```python
from build123d import *

# Parameters (mm, degrees)
SKETCH1_W              = 34
SKETCH1_H              = 150
BOSS_EXTRUDE1_DEPTH    = 6.35
SKETCH3_W              = 30
SKETCH3_H              = 6.35
BOSS_EXTRUDE2_DEPTH    = 6.35
F_8_CLEARANCE_HOLE1_D  = 4.3053
F_10_CLEARANCE_HOLE1_D = 4.9784


with BuildPart() as part:
    # Sketch1 → Boss-Extrude1 (new body)
    with BuildSketch(Plane.XY):
        Rectangle(SKETCH1_W, SKETCH1_H)
    extrude(amount=BOSS_EXTRUDE1_DEPTH)

    # Sketch3 → Boss-Extrude2 (add)
    with BuildSketch(Plane.XY.offset(6.35)):
        with Locations((0, 78.175)):
            Rectangle(SKETCH3_W, SKETCH3_H)
        with Locations((0, -78.175)):
            Rectangle(SKETCH3_W, SKETCH3_H)
    extrude(amount=-BOSS_EXTRUDE2_DEPTH)

    # #8 Clearance Hole1 (through all)
    with Locations(Plane.XY.offset(6.35)):
        with Locations((-8, 59.5), (8, 59.5), (8, 35.5), (-8, 35.5), (-8, -35.5), (-8, -59.5), (8, -59.5), (8, -35.5)):
            Hole(F_8_CLEARANCE_HOLE1_D / 2)

    # #10 Clearance Hole1 (through all)
    with Locations(Plane.XY.offset(6.35)):
        with Locations((-6.5, 10), (-6.5, -10)):
            Hole(F_10_CLEARANCE_HOLE1_D / 2)


solid = part.part
```
Work out the finished part from the listing and answer in its coordinate system (mm). A direction names the side the tool comes from. Round coordinates to 2 decimals unless told otherwise and drop trailing zeros. Write each loop counter-clockwise with the first axis right and the second up, starting at its lowest first coordinate (ties: lowest second). Pieces come first, ordered by that corner, then holes. Notation, with made-up numbers: (45.5, 52.5) -> (58.5, 52.5) arc R11 cw to (58.5, 57.5) -> close; hole circle Ø2 at (39, 60.25). An arc over 180 degrees is marked (long way). Write each question's results on one line, items separated by ' | '.
1) Which of the six approach directions +Z, -Z, +X, -X, +Y, -Y give full straight-line access (tool end or side, diameter ignored) to faces 1 (the flat face through (0, 1, 6.35)), 2 (the flat face through (-15, 78, 3)), 3 (the flat face through (15, -78, 3))?
Findings:
face 1: +Z, +X, -X, +Y, -Y | face 2: +Z, -Z, -X, +Y | face 3: +Z, -Z, +X, -Y
2) For a pull along X with two mould halves and no side action, classify faces 4 (the flat face through (15, 78, 3)), 5 (the flat face through (-15, -78, 3)), 6 (the cylindrical face through (5.947, -34.853, 3.131)), 7 (the flat face through (0, -81.35, 3)) as +X half, -X half, draft (parallel to the pull), parting line (faces both ways), or undercut.
Findings:
face 4: +X half | face 5: -X half | face 6: undercut | face 7: draft
3) The part is cut by section B-B (y = 59.5). Write down the section's boundary in (x, z), and give its area (3 significant figures).
Findings:
outline: (-17, 0) -> (-10.15, 0) -> (-10.15, 6.35) -> (-17, 6.35) -> close; (-5.85, 0) -> (5.85, 0) -> (5.85, 6.35) -> (-5.85, 6.35) -> close; (10.15, 0) -> (17, 0) -> (17, 6.35) -> (10.15, 6.35) -> close | area: 161 mm²
4) Consider line 1 along X through (y, z) = (-9, 4.75); line 2 along Y through (x, z) = (15.5, 6). Determine where each line is inside the solid, lowest interval first. Write a range as [from, to].
Findings:
line 1: x = [-17, -8.78], [-4.22, 17] | line 2: y = [-75, 75]
5) The part is cut by section C-C (z = 1.25). State how many separate pieces and enclosed holes the cut face has, and give its area (3 significant figures).
Findings:
separate pieces: 1 | enclosed holes: 10 | area: 5,330 mm²
6) Flat-ended cylindrical pins translate along their axes: pin 1 (2.5 mm diameter, centred on x = -8, y = 59.5, fed in from -Z); pin 2 (1 mm diameter, centred on x = -16, z = 3.5, fed in from +Y); pin 3 (1.9 mm diameter, centred on y = -77.5, z = 3, fed in from -X); pin 4 (3 mm diameter, centred on y = -79.5, z = 4.5, fed in from +X). Find the tip coordinate at first contact, or state that the pin passes through.
Findings:
pin 1: passes through | pin 2: stops at y = 75 | pin 3: stops at x = -15 | pin 4: stops at x = 15
7) The part is cut by section A-A (y = 10). Write down the section's boundary in (x, z).
Findings:
outline: (-17, 0) -> (-8.99, 0) -> (-8.99, 6.35) -> (-17, 6.35) -> close; (-4.01, 0) -> (17, 0) -> (17, 6.35) -> (-4.01, 6.35) -> close
